```python
from build123d import *

# Parameters (mm, degrees)
F0_W     = 127
F0_H     = 63.5
F1_DEPTH = 9.525
F3_D     = 9.8044
F5_D     = 6.5278


with BuildPart() as f1:
    # F0 (on Front) → F1 (new body, symmetric)
    with BuildSketch(Plane.XZ):
        Rectangle(F0_W, F0_H)
    extrude(amount=F1_DEPTH, both=True)

    # F3 (through all)
    with Locations(Plane.XZ.offset(9.525)):
        with Locations((-38.1, -6.35), (38.1, -6.35)):
            Hole(F3_D / 2)

    # F5 (through all)
    with Locations(Plane(origin=(0, 0, -31.75), x_dir=(1, 0, 0), z_dir=(0, 0, -1))):
        with Locations((-38.1, 0), (38.1, 0)):
            Hole(F5_D / 2)


solid = f1.part
```
The model under review builds one solid part; all positions refer to its coordinate system, in mm. Round coordinates to 2 decimals unless told otherwise and drop trailing zeros. Order: outer loops, then holes, each group sorted by start corner. A loop starts at its lowest first (then second) coordinate and runs counter-clockwise, first axis right, second up. Notation, with made-up numbers: (42, -13) -> (92, -13) arc R19 ccw to (92, 8) -> close; hole circle Ø4 at (-35, 79). An arc over 180 degrees is marked (long way). Use a Markdown table: item, result.
Q1. Mouldability with a two-part tool opening along X and no side actions: class faces 1 (the flat face through (-1, -9.525, 0)), 2 (the flat face through (-63.5, 0, 0)), 3 (the cylindrical face through (41.36, -0.14, 14.77)), 4 (the flat face through (63.5, 0, 0)) as +X half, -X half, draft (parallel to the pull), parting line (faces both ways), or undercut.
Values:
| item | result |
|---|---|
| face 1 | draft |
| face 2 | -X half |
| face 3 | undercut |
| face 4 | +X half |
Q2. We need section B-B on y = 0. Write out the cut boundary in (x, z).
Values:
| item | result |
|---|---|
| outline | (-63.5, -31.75) -> (-41.36, -31.75) -> (-41.36, -10.01) arc R4.9 cw to (-41.36, -2.69) -> (-41.36, 31.75) -> (-63.5, 31.75) -> close; (-34.84, -31.75) -> (34.84, -31.75) -> (34.84, -10.01) arc R4.9 cw to (34.84, -2.69) -> (34.84, 31.75) -> (-34.84, 31.75) -> (-34.84, -2.69) arc R4.9 cw to (-34.84, -10.01) -> close; (41.36, -31.75) -> (63.5, -31.75) -> (63.5, 31.75) -> (41.36, 31.75) -> (41.36, -2.69) arc R4.9 cw to (41.36, -10.01) -> close |
Q3. We need section D-D on z = -20.5. Write out the cut boundary in (x, y) (3 decimals), then the cut area to 3 significant figures.
Values:
| item | result |
|---|---|
| outline | (-63.5, -9.525) -> (63.5, -9.525) -> (63.5, 9.525) -> (-63.5, 9.525) -> close; hole circle Ø6.528 at (-38.1, 0); hole circle Ø6.528 at (38.1, 0) |
| area | 2,350 mm^2 |
Q4. For line 1 (X direction, y = -1.75, z = -6.5); line 2 (Y direction, x = -38.1, z = 9) (3 decimals); line 3 (X direction, y = 0.5, z = 21), list the stretches that pass through material, from the lowest coordinate up.
Values:
| item | result |
|---|---|
| line 1 | x = -63.5 to -43, -33.2 to 33.2, 43 to 63.5 |
| line 2 | y = -9.525 to -3.264, 3.264 to 9.525 |
| line 3 | x = -63.5 to -41.33, -34.87 to 34.87, 41.33 to 63.5 |
Q5. We need section C-C on z = -6.35. Write out the cut boundary in (x, y) (3 decimals).
Values:
| item | result |
|---|---|
| outline | (-63.5, -9.525) -> (-43.002, -9.525) -> (-43.002, 9.525) -> (-63.5, 9.525) -> close; (-33.198, -9.525) -> (33.198, -9.525) -> (33.198, 9.525) -> (-33.198, 9.525) -> close; (43.002, -9.525) -> (63.5, -9.525) -> (63.5, 9.525) -> (43.002, 9.525) -> close |
Q6. We need section A-A on x = -38.1. Write out the cut boundary in (y, z) (3 decimals), then the cut area to 3 significant figures.
Values:
| item | result |
|---|---|
| outline | (-9.525, -31.75) -> (-3.264, -31.75) -> (-3.264, -11.252) -> (-9.525, -11.252) -> close; (-9.525, -1.448) -> (-3.264, -1.448) -> (-3.264, 31.75) -> (-9.525, 31.75) -> close; (3.264, -31.75) -> (9.525, -31.75) -> (9.525, -11.252) -> (3.264, -11.252) -> close; (3.264, -1.448) -> (9.525, -1.448) -> (9.525, 31.75) -> (3.264, 31.75) -> close |
| area | 672 mm^2 |
